from build123d import *

# Parameters (mm, degrees)
SKETCH1_R           = 3
BOSS_EXTRUDE1_DEPTH = 5
SKETCH2_R           = 3
BOSS_EXTRUDE2_DEPTH = 5
SKETCH3_R           = 3
BOSS_EXTRUDE3_DEPTH = 10


with BuildPart() as part:
    # Sketch1 → Boss-Extrude1 (new body)
    with BuildSketch(Plane.XY):
        with BuildLine():
            Line((19.7, -5), (-19.7, -5))
            ThreePointArc((-19.7, -5), (-24.7, 0), (-19.7, 5))
            Line((-19.7, 5), (19.7, 5))
            ThreePointArc((19.7, 5), (24.7, 0), (19.7, -5))
        make_face()
        with Locations((19.7, 0)):
            Circle(SKETCH1_R, mode=Mode.SUBTRACT)
    extrude(amount=BOSS_EXTRUDE1_DEPTH)

    # Sketch2 → Boss-Extrude2 (add)
    with BuildSketch(Plane.XY.offset(5)):
        with Locations((-19.7, 0)):
            Circle(SKETCH2_R)
    extrude(amount=BOSS_EXTRUDE2_DEPTH)

    # Sketch3 → Boss-Extrude3 (add)
    with BuildSketch(Plane(origin=(0, 0, 0), x_dir=(-1, 0, 0), z_dir=(0, 0, -1))):
        with Locations((-19.7, 0)):
            Circle(SKETCH3_R)
    extrude(amount=-BOSS_EXTRUDE3_DEPTH)


solid = part.part
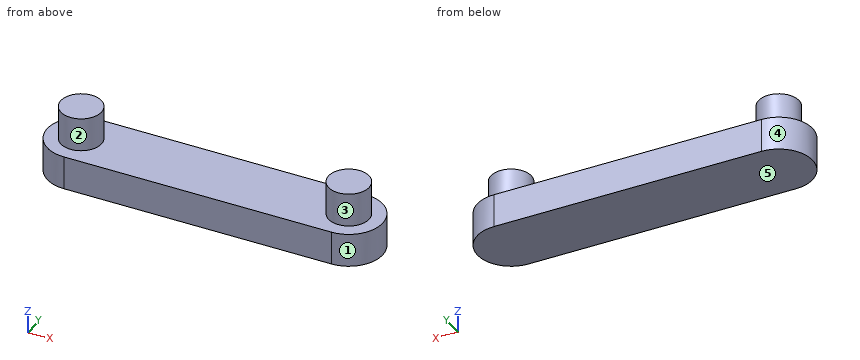
Read the model definition and answer for the solid it produces. Units are mm, in the model's axes. Face numbers are marked on the shaded views. A direction names the side the tool comes from. Round coordinates to 2 decimals unless told otherwise and drop trailing zeros. Order: outer loops, then holes, each group sorted by start corner. A loop starts at its lowest first (then second) coordinate and runs counter-clockwise, first axis right, second up. Notation, with made-up numbers: (-23, 49.5) - (-15, 49.5) arc R15 cw to (-15, 57.5) - close; hole circle Ø10 at (5, -11.75). An arc over 180 degrees is marked (long way). Use one line per item in the form item = value. Start each with the question number.
(1) The part is cut by section C-C (x = 9). Give the vertices of the cut face in (y, z), then the cut area to 3 significant figures.
(2) Flat-ended cylindrical pins translate along their axes: pin 1 Ø6 at (y, z) = (3, 8.5) entering from -X; pin 2 Ø3 at (x, y) = (-0.5, 2) entering from +Z. Find the tip coordinate at first contact, or state that the pin passes through.
(3) The part is cut by section A-A (y = 0). Give the vertices of the cut face in (x, z), then the cut area to 3 significant figures.
(4) For the marked faces 1 and 2, determine the directions among +Z, -Z, +X, -X, +Y, -Y from which every point of the face is accessible in a straight line to the end or side of a thin tool.
(5) Find the intervals of material crossed by line 1 along Z through (x, y) = (6, 1.75); line 2 along X through (y, z) = (-0.5, 7); line 3 along X through (y, z) = (1.75, 4.25), in increasing order. Write a range as from..to.
(6) Determine the mould class of the marked faces 3, 4 and 5 for opening direction X: +X half, -X half, draft (parallel to the pull), parting line (faces both ways), or undercut.
(7) The part is cut by section B-B (z = 9). Give the vertices of the cut face in (x, y), then the cut area to 3 significant figures.
(8) The part is cut by section D-D (z = 0.75). Give the vertices of the cut face in (x, y).
Checked values:
q1.outline = (-5, 0) - (5, 0) - (5, 5) - (-5, 5) - close
q1.area = 50.0 mm^2
q2.pin_1 = -22.7
q2.pin_2 = 5
q3.outline = (-24.7, 0) - (24.7, 0) - (24.7, 5) - (22.7, 5) - (22.7, 10) - (16.7, 10) - (16.7, 5) - (-16.7, 5) - (-16.7, 10) - (-22.7, 10) - (-22.7, 5) - (-24.7, 5) - close
q3.area = 307 mm^2
q4.face_1 = +Z, -Z, +X
q4.face_2 = +Z
q5.line_1 = 0..5
q5.line_2 = -22.66..-16.74, 16.74..22.66
q5.line_3 = -24.38..24.38
q6.face_3 = undercut
q6.face_4 = -X half
q6.face_5 = draft
q7.outline = circle Ø6 at (-19.7, 0); circle Ø6 at (19.7, 0)
q7.area = 56.5 mm^2
q8.outline = (-19.7, -5) - (19.7, -5) arc R5 ccw to (19.7, 5) - (-19.7, 5) arc R5 ccw to start
